For this review, take the finished solid that the model builds, in its own axes (mm). Coordinates: 2 decimals unless noted, no trailing zeros. Write each loop counter-clockwise with the first axis right and the second up, starting at its lowest first coordinate (ties: lowest second). Pieces come first, ordered by that corner, then holes.
1) We need section B-B on z = 350. Write out the cut boundary in (x, y).
2) To check wall thickness, follow line 1 along Y through (x, z) = (0.4, 350); line 2 along X through (y, z) = (-29.25, 272.5); line 3 along Y through (x, z) = (6.5, 272.5). State the ranges of each line that lie inside material, in increasing order.
3) Insertion check: P1, Ø9.5, axis at y = -22, z = 275, coming from the +X side; P2, Ø2, axis at x = 12, z = 208, coming from the +Y side; P3, Ø6.5, axis at y = -24.89, z = 10, coming from the -X side. Each pin has a flat end and moves straight along its axis. Give the tip position at first contact, or say it passes through.
4) We need section A-A on z = 126. Write out the cut boundary in (x, y), then the cut area to 3 significant figures.
5) We need section C-C on x = 10. Write out the cut boundary in (y, z).
from build123d import *

# Parameters (mm, degrees)
BOSS_EXTRUDE1_DEPTH = 380
SKETCH2_R           = 2
CUT_EXTRUDE1_DEPTH  = 10
CUT_EXTRUDE2_DEPTH  = 10
SKETCH5_R           = 5
CUT_EXTRUDE3_DEPTH  = 10
LPATTERN1_COUNT     = 21
LPATTERN1_PITCH     = 16
FILLET1_R           = 10


with BuildPart() as part:
    # Sketch1 → Boss-Extrude1 (new body)
    with BuildSketch(Plane.XY):
        Polygon((0, -15.388010819), (0, -35.388010819), (20, -35.388010819), (20, -34.388010819), (1, -34.388010819), (1, -15.388010819), align=None)
    extrude(amount=BOSS_EXTRUDE1_DEPTH)

    # Sketch2 → Cut-Extrude1 (cut)
    with BuildSketch(Plane(origin=(1, 0, 0), x_dir=(0, 0, -1), z_dir=(1, 0, 0))):
        with Locations(Location((-10, -24.888010819, 0), (0, 0, 90))):
            Circle(SKETCH2_R)
        with Locations(Location((-370, -24.888010819, 0), (0, 0, 90))):
            Circle(SKETCH2_R)
    extrude(amount=-CUT_EXTRUDE1_DEPTH, mode=Mode.SUBTRACT)

    # Sketch4 → Cut-Extrude2 (cut)
    with BuildSketch(Plane(origin=(0, -34.388010819, 0), x_dir=(1, 0, 0), z_dir=(0, 1, 0))):
        Polygon((1, 0), (16, -115), (16, -155), (1, -380), (1, -389.212459491), (24.909334079, -389.212459491), (24.909334079, 2.402258562), (1, 2.402258562), align=None)
    extrude(amount=-CUT_EXTRUDE2_DEPTH, mode=Mode.SUBTRACT)

    # Sketch5 → Cut-Extrude3 (cut)
    with BuildSketch(Plane(origin=(1, 0, 0), x_dir=(0, 0, -1), z_dir=(1, 0, 0))):
        with Locations(Location((-350, -24.888010819, 0), (0, 0, 90))):
            Circle(SKETCH5_R)
    cut_extrude3 = extrude(amount=-CUT_EXTRUDE3_DEPTH, mode=Mode.SUBTRACT)

    # LPattern1: Cut-Extrude3 ×21
    with Locations(*[(0, 0, -i * LPATTERN1_PITCH) for i in range(1, LPATTERN1_COUNT)]):
        add(cut_extrude3, mode=Mode.SUBTRACT)

    # Fillet1
    fillet1_edges = [part.edges().sort_by_distance(p)[0] for p in [
        (0.5, -15.388010819, 380),
        (0.5, -15.388010819, 0),
    ]]
    fillet(fillet1_edges, radius=FILLET1_R)


solid = part.part
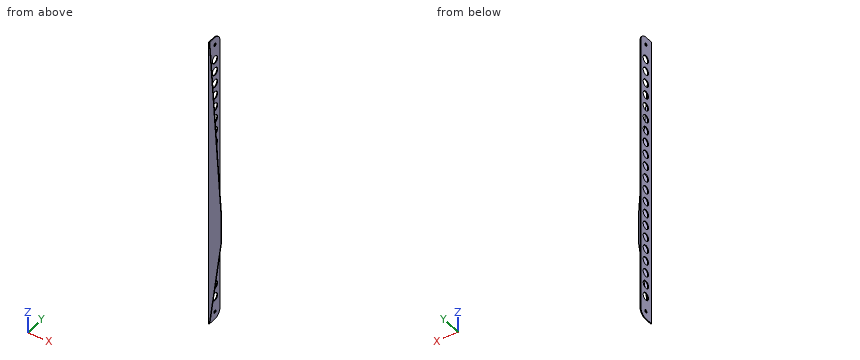
Result:
1. outline: (0, -35.39) - (3, -35.39) - (3, -34.39) - (1, -34.39) - (1, -29.89) - (0, -29.89) - close; (0, -19.89) - (1, -19.89) - (1, -15.39) - (0, -15.39) - close
2. line 1: y = -35.39 to -29.89, -19.89 to -15.39
2. line 2: x = 0 to 1
2. line 3: y = -35.39 to -34.39
3. P1: stops at x = 1
3. P2: stops at y = -34.39
3. P3: stops at x = 0
4. outline: (0, -35.39) - (16, -35.39) - (16, -34.39) - (1, -34.39) - (1, -29.89) - (0, -29.89) - close; (0, -19.89) - (1, -19.89) - (1, -15.39) - (0, -15.39) - close
4. area: 25.0 mm2
5. outline: (-35.39, 69) - (-34.39, 69) - (-34.39, 245) - (-35.39, 245) - close
